Read the model definition and answer for the solid it produces. Units are mm, in the model's axes. A direction names the side the tool comes from. Round coordinates to 2 decimals unless told otherwise and drop trailing zeros. Order: outer loops, then holes, each group sorted by start corner. A loop starts at its lowest first (then second) coordinate and runs counter-clockwise, first axis right, second up. Notation, with made-up numbers: M -19.75,-19.75 L 21.25,-19.75 A10 cw 21.25,-7.75 Z; hole C 46.5,-1.75 d6. An arc over 180 degrees is marked long. Answer as CSV lines item,"result".
```python
from build123d import *

# Parameters (mm, degrees)
SKETCH1_W           = 19
SKETCH1_H           = 6.3
BOSS_EXTRUDE1_DEPTH = 1
SKETCH1_3_W         = 4.6
SKETCH1_3_H         = 4.6
BOSS_EXTRUDE2_DEPTH = 9.4
FILLET6_R           = 1
FILLET7_R           = 1
FILLET9_R           = 0.5
FILLET10_R          = 0.5
CUT_EXTRUDE6_DEPTH  = 3


with BuildPart() as part:
    # Sketch1 → Boss-Extrude1 (new body)
    with BuildSketch(Plane(origin=(0, 0, 0), x_dir=(1, 0, 0), z_dir=(0, 1, 0))):
        with Locations((2.580402043, 0.806197617)):
            Rectangle(SKETCH1_W, SKETCH1_H)
    extrude(amount=BOSS_EXTRUDE1_DEPTH)

    # Sketch1_3 → Boss-Extrude2 (add)
    with BuildSketch(Plane(origin=(0, 0, 0), x_dir=(1, 0, 0), z_dir=(0, 1, 0))):
        with Locations((2.580402043, 0.806197617)):
            Rectangle(SKETCH1_3_W, SKETCH1_3_H)
    extrude(amount=BOSS_EXTRUDE2_DEPTH)

    # Fillet6
    fillet6_edges = [part.edges().sort_by_distance(p)[0] for p in [
        (4.880402043, 9.4, -0.806197617),
    ]]
    fillet(fillet6_edges, radius=FILLET6_R)

    # Fillet7
    fillet7_edges = [part.edges().sort_by_distance(p)[0] for p in [
        (0.280402043, 9.4, -0.806197617),
    ]]
    fillet(fillet7_edges, radius=FILLET7_R)

    # Fillet9
    fillet9_edges = [part.edges().sort_by_distance(p)[0] for p in [
        (4.880402043, 1, -0.806197617),
    ]]
    fillet(fillet9_edges, radius=FILLET9_R)

    # Fillet10
    fillet10_edges = [part.edges().sort_by_distance(p)[0] for p in [
        (0.280402043, 1, -0.806197617),
    ]]
    fillet(fillet10_edges, radius=FILLET10_R)

    # Sketch1_6 → Cut-Extrude6 (cut)
    with BuildSketch(Plane(origin=(0, 0, 0), x_dir=(1, 0, 0), z_dir=(0, 1, 0))):
        Polygon((3.330402043, 0.525612743), (3.330402043, 1.096346732), (3.430402043, 1.096346732), (3.430402043, 1.656197617), (2.868074208, 1.656197617), (2.868074208, 1.556197617), (2.282451593, 1.556197617), (2.282451593, 1.656197617), (1.730402043, 1.656197617), (1.730402043, 1.096346732), (1.830402043, 1.096346732), (1.830402043, 0.525612743), (1.730402043, 0.525612743), (1.730402043, -0.043802383), (2.321489292, -0.043802383), (2.321489292, 0.056197617), (2.868074208, 0.056197617), (2.868074208, -0.043802383), (3.430402043, -0.043802383), (3.430402043, 0.525612743), align=None)
    extrude(amount=CUT_EXTRUDE6_DEPTH, mode=Mode.SUBTRACT)


solid = part.part
```
Item 1: Determine the mould class of faces 4 (the face through (2, 0, 1)), 5 (the face through (4.595, 9.099, -0.838)), 6 (the face through (3, 3, -1)) for opening direction X: +X half, -X half, draft (parallel to the pull), parting line (faces both ways), or undercut.
Ans:
face 4,"draft"
face 5,"+X half"
face 6,"undercut"
Item 2: A cutting plane is placed at D-D, the plane y = 7.75. Determine the outline of the cut face in (x, z), and give its area (3 significant figures).
Ans:
outline,"M 0.28,-3.11 L 4.88,-3.11 L 4.88,1.49 L 0.28,1.49 Z"
area,"21.2 mm2"
Item 3: A cutting plane is placed at C-C, the plane x = 0.5. Determine the outline of the cut face in (y, z), and give its area (3 significant figures).
Ans:
outline,"M 0,-3.96 L 1,-3.96 L 1,-3.11 L 9.03,-3.11 L 9.03,1.49 L 1,1.49 L 1,2.34 L 0,2.34 Z"
area,"43.2 mm2"
Item 4: A cutting plane is placed at B-B, the plane z = 0.25. Determine the outline of the cut face in (x, y).
Ans:
outline,"M -6.92,0 L 12.08,0 L 12.08,1 L 5.38,1 A0.5 cw 4.88,1.5 L 4.88,8.4 A1 ccw 3.88,9.4 L 1.28,9.4 A1 ccw 0.28,8.4 L 0.28,1.5 A0.5 cw -0.22,1 L -6.92,1 Z"
Item 5: Flat-ended cylindrical pins translate along their axes: pin 1 (0.5 mm diameter, centred on x = 2, y = 1.5, fed in from -Z); pin 2 (0.5 mm diameter, centred on y = 2, z = 0, fed in from +X); pin 3 (0.6 mm diameter, centred on y = 1.5, z = -0.5, fed in from -X). Find the tip coordinate at first contact, or state that the pin passes through.
Ans:
pin 1,"z = -3.11"
pin 2,"x = 4.88"
pin 3,"x = 0.18"
Item 6: A cutting plane is placed at A-A, the plane y = 1.75. Determine the outline of the cut face in (x, z).
Ans:
outline,"M 0.28,-3.11 L 4.88,-3.11 L 4.88,1.49 L 0.28,1.49 Z; hole M 1.73,-1.66 L 2.28,-1.66 L 2.28,-1.56 L 2.87,-1.56 L 2.87,-1.66 L 3.43,-1.66 L 3.43,-1.1 L 3.33,-1.1 L 3.33,-0.53 L 3.43,-0.53 L 3.43,0.04 L 2.87,0.04 L 2.87,-0.06 L 2.32,-0.06 L 2.32,0.04 L 1.73,0.04 L 1.73,-0.53 L 1.83,-0.53 L 1.83,-1.1 L 1.73,-1.1 Z"
Item 7: Find the intervals of material crossed by probe 1 along X at (y, z) = (1.75, -1); probe 2 along Y at (x, z) = (-3.25, 1); probe 3 along X at (y, z) = (5.5, -0.5), in increasing order. Write a range as [from, to].
Ans:
probe 1,"[0.28, 1.83], [3.33, 4.88]"
probe 2,"[0, 1]"
probe 3,"[0.28, 4.88]"
Item 8: A tool of negligible diameter and unlimited length cuts with its end or side. For faces 1 (the face through (0.28, 5, -1)), 2 (the face through (4.88, 5, -1)), 3 (the face through (3, 5, 1.494)), from which of +Z, -Z, +X, -X, +Y, -Y can it reach the whole face along a straight path? Write none if from no direction.
Ans:
face 1,"+Z, -Z, -X, +Y"
face 2,"+Z, -Z, +X, +Y"
face 3,"+Z, +X, -X, +Y"
